```python
from build123d import *

# Parameters (mm, degrees)
SKETCH_13_W           = 41
SKETCH_13_H           = 38
BOSS_EXTRUDE1_DEPTH   = 14
BOSS_EXTRUDE1_2_DEPTH = 14
SKETCH1_R             = 31
SKETCH1_R_2           = 10
BOSS_EXTRUDE2_DEPTH   = 25


with BuildPart() as part:
    # Эскиз13 → Boss-Extrude1 (new body)
    with BuildSketch(Plane(origin=(0, -36, 0), x_dir=(-1, 0, 0), z_dir=(0, 1, 0))):
        with Locations((-7.5, 17.5)):
            Rectangle(SKETCH_13_W, SKETCH_13_H)
    extrude(amount=BOSS_EXTRUDE1_DEPTH)



with BuildPart() as body_2:
    # Эскиз13 → Boss-Extrude1 2 (new body)
    with BuildSketch(Plane(origin=(0, -36, 0), x_dir=(-1, 0, 0), z_dir=(0, 1, 0))):
        with Locations((-92.5, 17.5)):
            Rectangle(SKETCH_13_W, SKETCH_13_H)
    extrude(amount=BOSS_EXTRUDE1_2_DEPTH)


with BuildPart() as part_1:
    add(part.part)

    add(body_2.part)  # Boss-Extrude2 merges body 2
    # Sketch1 → Boss-Extrude2 (add)
    with BuildSketch(Plane.XY.offset(5)):
        with Locations((50, -1.5)):
            Circle(SKETCH1_R)
        with Locations((50, -1.5)):
            Circle(SKETCH1_R_2, mode=Mode.SUBTRACT)
    extrude(amount=BOSS_EXTRUDE2_DEPTH)


solid = part_1.part
```
CAD build for the part. Positions are in the model's coordinates, mm. Round coordinates to 2 decimals unless told otherwise and drop trailing zeros. Write each loop counter-clockwise with the first axis right and the second up, starting at its lowest first coordinate (ties: lowest second). Pieces come first, ordered by that corner, then holes.
Item 1: Drop flat-ended pins along their axis: pin 1 Ø4 at (x, z) = (37.5, 13.5) entering from +Y; pin 2 Ø4 at (x, z) = (7.5, 20) entering from +Y; pin 3 Ø10 at (x, y) = (77, 1) entering from +Z. Give the stop position or say it passes through.
Filled in:
pin 1: stops at y = 27.67
pin 2: stops at y = -22
pin 3: stops at z = 30
Item 2: Band-saw the part on A-A on x = 50. Write the cut outline in (y, z).
Filled in:
outline: (-32.5, 5) - (-11.5, 5) - (-11.5, 30) - (-32.5, 30) - close; (8.5, 5) - (29.5, 5) - (29.5, 30) - (8.5, 30) - close
Item 3: Band-saw the part on B-B on y = -1.5. Write the cut outline in (x, z), then the cut area to 3 significant figures.
Filled in:
outline: (19, 5) - (40, 5) - (40, 30) - (19, 30) - close; (60, 5) - (81, 5) - (81, 30) - (60, 30) - close
area: 1,050 mm2
Item 4: Band-saw the part on D-D on x = 29.5. Write the cut outline in (y, z), then the cut area to 3 significant figures.
Filled in:
outline: (-24.75, 5) - (21.75, 5) - (21.75, 30) - (-24.75, 30) - close
area: 1,160 mm2
Item 5: Mould opens along X. For faces 1 (the flat face through (113, -29, 17)), 2 (the flat face through (28, -29, 17)), 3 (the flat face through (8, -29, -1.5)) say: released by +X, released by -X, zero draft, split by the parting line, or undercut.
Filled in:
face 1: released by +X
face 2: undercut
face 3: zero draft
Item 6: Band-saw the part on C-C on y = -26. Write the cut outline in (x, z).
Filled in:
outline: (-13, -1.5) - (28, -1.5) - (28, 36.5) - (-13, 36.5) - close; (31.01, 5) - (68.99, 5) - (68.99, 30) - (31.01, 30) - close; (72, -1.5) - (113, -1.5) - (113, 36.5) - (72, 36.5) - close
Item 7: Drill centre lines: L1, parallel to Y at x = 50, z = 12; L2, parallel to X at y = -1, z = 24; L3, parallel to Y at x = 1.5, z = 0.5. Where is each one in solid material? Low to high.
Filled in:
L1: y = -32.5 to -11.5, 8.5 to 29.5
L2: x = 19 to 40.01, 59.99 to 81
L3: y = -36 to -22
